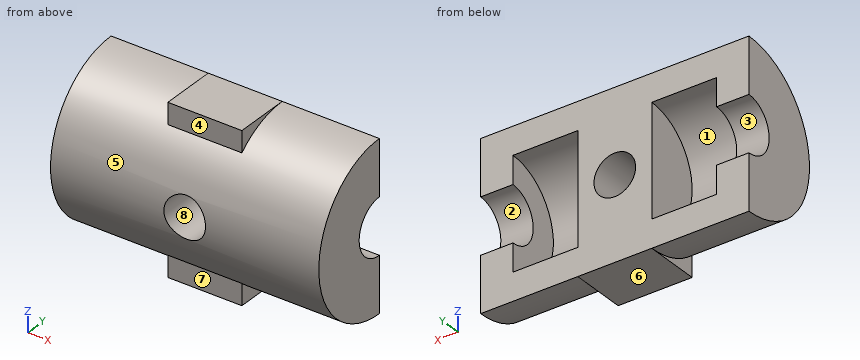
```python
from build123d import *

# Parameters (mm, degrees)
CUT_EXTRUDE1_DEPTH      = 10
CUT_EXTRUDE1_DEPTH_BACK = 10
SKETCH4_R               = 2.25
SKETCH4_3_W             = 8
SKETCH4_3_H             = 18
SKETCH4_3_R             = 2.25
BOSS_EXTRUDE1_DEPTH     = 6
CUT_EXTRUDE2_DEPTH      = 32.670175393
CUT_EXTRUDE2_DEPTH_BACK = 32.670175393


with BuildPart() as part:
    # Sketch1 → Revolve1 (revolve)
    with BuildSketch(Plane.XY, mode=Mode.PRIVATE) as revolve1_sk:
        Polygon((-14.5, 9), (14.5, 9), (14.5, 3), (11, 3), (11, 6), (-11, 6), (-11, 3), (-14.5, 3), align=None)
    revolve(revolve1_sk.sketch.rotate(Axis((-39.087837838, 0, 0), (1, 0, 0)), 90), axis=Axis((-39.087837838, 0, 0), (1, 0, 0)))

    # Sketch4 → Cut-Extrude1 (cut, two sides: drawn at the far end of the back side and taken through both)
    with BuildSketch(Plane(origin=(0, 0, 0), x_dir=(1, 0, 0), z_dir=(0, 1, 0)).offset(-CUT_EXTRUDE1_DEPTH_BACK)):
        with Locations(Location((0, 0, 0), (0, 0, 90))):
            Circle(SKETCH4_R)
    extrude(amount=CUT_EXTRUDE1_DEPTH + CUT_EXTRUDE1_DEPTH_BACK, mode=Mode.SUBTRACT)

    # Sketch4_3 → Boss-Extrude1 (add, symmetric)
    with BuildSketch(Plane(origin=(0, 0, 0), x_dir=(1, 0, 0), z_dir=(0, 1, 0))):
        Rectangle(SKETCH4_3_W, SKETCH4_3_H)
        with Locations(Location((0, 0, 0), (0, 0, 90))):
            Circle(SKETCH4_3_R, mode=Mode.SUBTRACT)
    extrude(amount=BOSS_EXTRUDE1_DEPTH, both=True)

    # Sketch5 → Cut-Extrude2 (cut, two sides: drawn at the far end of the back side and taken through both)
    with BuildSketch(Plane.ZY.offset(14.5).offset(-CUT_EXTRUDE2_DEPTH_BACK)):
        Polygon((-61.985560785, 0), (-9.284472497, 0), (10.360933076, 0), (63.062021365, 0), (63.062021365, 105.402176578), (-61.985560785, 105.402176578), align=None)
    extrude(amount=CUT_EXTRUDE2_DEPTH + CUT_EXTRUDE2_DEPTH_BACK, mode=Mode.SUBTRACT)


solid = part.part
```
Part model, mm, in its own coordinate system. Face numbers are marked on the shaded views. A direction names the side the tool comes from. Round coordinates to 2 decimals unless told otherwise and drop trailing zeros. Write each loop counter-clockwise with the first axis right and the second up, starting at its lowest first coordinate (ties: lowest second). Pieces come first, ordered by that corner, then holes.
Item 1: Cut at A-A, the plane z = 0. Give the cut face in (x, y), plus the area to 4 significant figures.
Results:
outline: (-14.5, -9) - (-2.25, -9) - (-2.25, 0) - (-4, 0) - (-4, -6) - (-11, -6) - (-11, -3) - (-14.5, -3) - close; (2.25, -9) - (14.5, -9) - (14.5, -3) - (11, -3) - (11, -6) - (4, -6) - (4, 0) - (2.25, 0) - close
area: 115.5 mm2
Item 2: Which spindle directions (+Z, -Z, +X, -X, +Y, -Y) get a long thin tool onto all of the face, cutting with end or side? Do the marked faces 1, 2, 3, 4 and 5. Say none if no direction does.
Results:
face 1: +Y
face 2: +X, +Y
face 3: -X, +Y
face 4: +Z, +X, -X, -Y
face 5: -Y
Item 3: Cut at B-B, the plane x = 0. Give the cut face in (y, z).
Results:
outline: (-8.71, -2.25) arc R9 ccw to (-6, -6.71) - (-6, -9) - (0, -9) - (0, -2.25) - close; (-8.71, 2.25) - (0, 2.25) - (0, 9) - (-6, 9) - (-6, 6.71) arc R9 ccw to start
Item 4: Two-plate mould, pull along Z, no slides. Class the marked faces 6, 7 and 8: +Z half, -Z half, draft (parallel to the pull), parting line (faces both ways), or undercut.
Results:
face 6: -Z half
face 7: draft
face 8: undercut
Item 5: Drop a flat-ended pin along its axis: pin 1 Ø0.7 at (x, z) = (1.5, 7.5) entering from -Y. Give the stop position or say it passes through.
Results:
pin 1: stops at y = -6
Item 6: Probe L1, parallel to X at y = -4, z = 0; L2, parallel to X at y = -3, z = 5; L3, parallel to X at y = -2, z = 0. List the from-to ranges inside material, lowest first.
Results:
L1: x = -14.5 to -11, -4 to -2.25, 2.25 to 4, 11 to 14.5
L2: x = -14.5 to -11, -4 to 4, 11 to 14.5
L3: x = -4 to -2.25, 2.25 to 4
Item 7: Cut at D-D, the plane x = -3.5. Give the cut face in (y, z), plus the area to 3 significant figures.
Results:
outline: (-6, -9) - (0, -9) - (0, 9) - (-6, 9) - (-6, 6.71) arc R9 ccw to (-6, -6.71) - close
area: 136 mm2
